Read the model definition and answer for the solid it produces. Units are mm, in the model's axes. Coordinates: 2 decimals unless noted, no trailing zeros. Order: outer loops, then holes, each group sorted by start corner. A loop starts at its lowest first (then second) coordinate and runs counter-clockwise, first axis right, second up. Notation, with made-up numbers: (51, 4) -> (70, 4) arc R7 cw to (70, 16) -> close; hole circle Ø2 at (53, -22). An arc over 180 degrees is marked (long way). Return JSON: item names as keys, results as strings. Group by question number.
```python
from build123d import *

# Parameters (mm, degrees)
SKETCH_1_R             = 5.25
SKETCH_1_R_2           = 30
SM_BASE_FLANGE_1_DEPTH = 6


# Sheet-metal steps are written as plain solids
with BuildPart() as part:
    # Sketch 1 → Базовая кромка1 (new body)
    with BuildSketch(Plane.XY):
        with BuildLine():
            Line((0.033417561, 126.694802442), (-68.913342264, 27.562479168))
            ThreePointArc((-68.913342264, 27.562479168), (-68.526745087, 24.270869385), (-65.212546165, 24.255447089))
            ThreePointArc((-65.212546165, 24.255447089), (-54.703732736, 27.822860554), (-44.750337246, 22.914549568))
            ThreePointArc((-44.750337246, 22.914549568), (-39.302081877, 13.457030285), (-37.908757817, 2.63174481))
            ThreePointArc((-37.908757817, 2.63174481), (-35.176905519, -14.373076153), (-25.219001767, -28.425375105))
            ThreePointArc((-25.219001767, -28.425375105), (96.595176943, -66.317354816), (205.574554402, 0))
            ThreePointArc((205.574554402, 0), (67.691260765, -15.667826508), (22.08143844, 115.393333105))
            ThreePointArc((22.08143844, 115.393333105), (15.997331025, 130.681317743), (0.033417561, 126.694802442))
        make_face()
        with Locations((10.295453487, 119.557532751)):
            Circle(SKETCH_1_R, mode=Mode.SUBTRACT)
        Circle(SKETCH_1_R_2, mode=Mode.SUBTRACT)
    extrude(amount=-SM_BASE_FLANGE_1_DEPTH)


solid = part.part
```
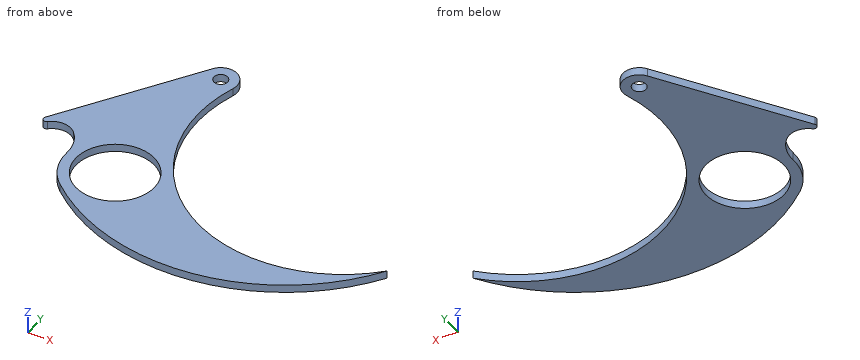
1. Given pin 1 (2 mm diameter, centred on y = -39, z = -5, fed in from +X); pin 2 (3 mm diameter, centred on x = 27.5, z = -1, fed in from +Y), each flat-ended and moving along its own axis, determine where each tip first touches the part or whether it passes through.
2. Find section B-B on y = 14.5. Determine the outline of the cut face in (x, z).
3. Find section C-C on x = 113. Determine the outline of the cut face in (y, z).
4. Find section D-D on y = 108.5. Determine the outline of the cut face in (x, z), and give its area (3 significant figures).
5. Straight lines are drawn through the part: L1, parallel to Y at x = -8, z = -5.15; L2, parallel to Y at x = 7.5, z = -0.3; L3, parallel to Y at x = -25, z = -4.65. For each, find the intervals that lie inside material, in ascending order.
6. Find section A-A on z = -3.8. Determine the outline of the cut face in (x, y).
Result:
{
 "1": {"pin 1": "x = 168.59", "pin 2": "y = 31.74"},
 "2": {"outline": "(-39.68, -6) -> (-26.26, -6) -> (-26.26, 0) -> (-39.68, 0) -> close; (26.26, -6) -> (35.94, -6) -> (35.94, 0) -> (26.26, 0) -> close"},
 "3": {"outline": "(-63.39, -6) -> (-31.85, -6) -> (-31.85, 0) -> (-63.39, 0) -> close"},
 "4": {"outline": "(-12.62, -6) -> (19.9, -6) -> (19.9, 0) -> (-12.62, 0) -> close", "area": "195 mm^2"},
 "5": {"L1": "-41.67 to -28.91, 28.91 to 115.14", "L2": "-50.7 to -29.05, 29.05 to 115.11, 124 to 131.74", "L3": "-28.62 to -16.58, 16.58 to 90.7"},
 "6": {"outline": "(-68.91, 27.56) arc R2.5 ccw to (-65.21, 24.26) arc R14.5 cw to (-44.75, 22.91) arc R27.84 cw to (-37.91, 2.63) arc R38 ccw to (-25.22, -28.43) arc R155 ccw to (205.57, 0) arc R111.1 cw to (22.08, 115.39) arc R12.5 ccw to (0.03, 126.69) -> close; hole circle Ø60 at (0, 0); hole circle Ø10.5 at (10.3, 119.56)"}
}
